Geometry check sheet. Reference: the model listing, model coordinates, mm. Face numbers are marked on the shaded views. A direction names the side the tool comes from. Round coordinates to 2 decimals unless told otherwise and drop trailing zeros. Write each loop counter-clockwise with the first axis right and the second up, starting at its lowest first coordinate (ties: lowest second). Pieces come first, ordered by that corner, then holes. Notation, with made-up numbers: (35.25, 54.25) - (83.25, 54.25) arc R10 cw to (83.25, 59.25) - close; hole circle Ø8 at (42, 16). An arc over 180 degrees is marked (long way). Return JSON: item names as keys, results as strings.
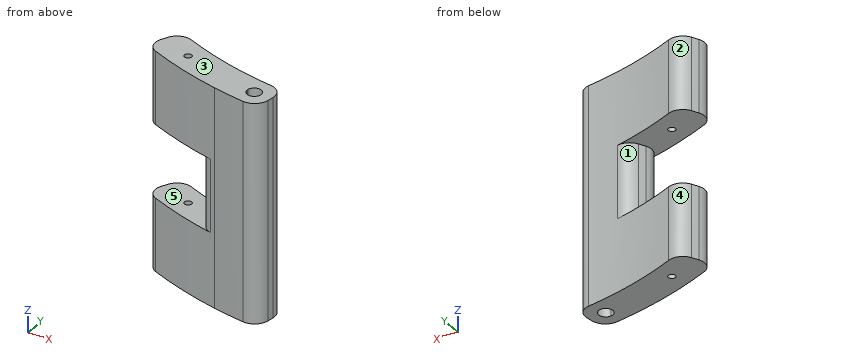
```python
from build123d import *

# Parameters (mm, degrees)
BOSS_EXTRUDE1_DEPTH     = 30
SKETCH2_W               = 10
SKETCH2_H               = 10
CUT_EXTRUDE2_DEPTH      = 37.330733855
SKETCH3_R               = 0.5
CUT_EXTRUDE3_DEPTH      = 30
FILLET1_R               = 2
SKETCH4_W               = 30
SKETCH4_H               = 5
BOSS_EXTRUDE2_DEPTH     = 10
FILLET2_R               = 2
FILLET3_R               = 2
CUT_EXTRUDE4_DEPTH      = 80.110177146
SKETCH6_W               = 10
SKETCH6_H               = 6
SKETCH8_W               = 10
SKETCH8_H               = 2.121165988
CUT_EXTRUDE5_DEPTH      = 80.110177146
FILLET4_R               = 8
CUT_EXTRUDE6_DEPTH      = 80.110177146
CUT_EXTRUDE6_DEPTH_BACK = 50
SCALE1_SCALE            = 1.9329
SCALE2_SCALE            = 1.5
CUT_EXTRUDE7_DEPTH      = 134.461525953
CUT_EXTRUDE7_DEPTH_BACK = 134.461525953
SKETCH10_R              = 280.344567012
SKETCH10_R_2            = 173.961
FILLET5_R               = 6


with BuildPart() as part:
    # Sketch1 → Boss-Extrude1 (new body)
    with BuildSketch(Plane.XY):
        with BuildLine():
            Line((-24.447759697, -49.267707941), (-26.670283306, -53.746590482))
            ThreePointArc((-26.670283306, -53.746590482), (-17.396934794, -57.422527459), (-7.642718065, -59.511249866))
            Line((-7.642718065, -59.511249866), (-7.005824893, -54.551979044))
            ThreePointArc((-7.005824893, -54.551979044), (-15.947190228, -52.637316837), (-24.447759697, -49.267707941))
        make_face()
    extrude(amount=BOSS_EXTRUDE1_DEPTH)

    # Sketch2 → Cut-Extrude2 (cut, through all)
    with BuildSketch(Plane(origin=(-26.670283306, -53.746590482, 0), x_dir=(0, 0, -1), z_dir=(0.4445047217595844, 0.8957765080272169, 0))):
        with Locations((-15, -5)):
            Rectangle(SKETCH2_W, SKETCH2_H)
    extrude(amount=CUT_EXTRUDE2_DEPTH, mode=Mode.SUBTRACT)

    # Sketch3 → Cut-Extrude3 (cut)
    with BuildSketch(Plane.XY.offset(30)):
        with Locations((-20.983324138, -53.534569281)):
            Circle(SKETCH3_R)
    extrude(amount=-CUT_EXTRUDE3_DEPTH, mode=Mode.SUBTRACT)

    # Fillet1
    fillet1_edges = [part.edges().sort_by_distance(p)[0] for p in [
        (-26.670283306, -53.746590482, 5),
        (-24.447759697, -49.267707941, 5),
        (-15.082503417, -52.891569183, 15),
        (-17.339488899, -57.439900111, 15),
        (-26.670283306, -53.746590482, 25),
        (-24.447759697, -49.267707941, 25),
    ]]
    fillet(fillet1_edges, radius=FILLET1_R)

    # Sketch4 → Boss-Extrude2 (add)
    with BuildSketch(Plane(origin=(-7.515339431, -58.519395701, 0), x_dir=(0, 0, -1), z_dir=(-0.12737863441697944, -0.9918541644284535, 0))):
        with Locations((-15, -2.5)):
            Rectangle(SKETCH4_W, SKETCH4_H)
    extrude(amount=BOSS_EXTRUDE2_DEPTH)

    # Fillet2
    fillet2_edges = [part.edges().sort_by_distance(p)[0] for p in [
        (-12.575405439, -58.667360415, 15),
    ]]
    fillet(fillet2_edges, radius=FILLET2_R)

    # Fillet3
    fillet3_edges = [part.edges().sort_by_distance(p)[0] for p in [
        (-7.005824893, -54.551979044, 15),
    ]]
    fillet(fillet3_edges, radius=FILLET3_R)

    # Sketch5 → Cut-Extrude4 (cut, through all)
    with BuildSketch(Plane.XY.offset(30)):
        with BuildLine():
            ThreePointArc((-10.9503146, -65.639855348), (-11.509930999, -66.072093113), (-11.077693234, -66.631709513))
            Line((-11.077693234, -66.631709513), (-10.9503146, -65.639855348))
        make_face()
        with BuildLine():
            Line((-10.9503146, -65.639855348), (-11.077693234, -66.631709513))
            ThreePointArc((-11.077693234, -66.631709513), (-10.683734829, -66.51117866), (-10.514003917, -66.135782431))
            ThreePointArc((-10.514003917, -66.135782431), (-10.638607687, -65.805513342), (-10.9503146, -65.639855348))
        make_face()
    extrude(amount=-CUT_EXTRUDE4_DEPTH, mode=Mode.SUBTRACT)

    # Cut-Sweep1: sweep along a path in Sketch7
    with BuildLine(Plane.XY) as cut_sweep1_path:
        Line((-8.024853968, -62.486812359), (-12.806249613, -60.46486559))
    # Sketch6 → Cut-Sweep1 (sweep, cut)
    with BuildSketch(Plane(origin=(0, 0, 0), x_dir=(0, 0, -1), z_dir=(0.9918541644284535, -0.1273786344169795, 0))):
        with Locations((-15, -66)):
            Rectangle(SKETCH6_W, SKETCH6_H)
    sweep(path=cut_sweep1_path.line, mode=Mode.SUBTRACT)

    # Sketch8 → Cut-Extrude5 (cut, through all)
    with BuildSketch(Plane(origin=(0, 0, 0), x_dir=(0, 0, -1), z_dir=(0.9918541644284535, -0.1273786344169795, 0))):
        with Locations((-15, -67.939417006)):
            Rectangle(SKETCH8_W, SKETCH8_H)
    extrude(amount=-CUT_EXTRUDE5_DEPTH, mode=Mode.SUBTRACT)

    # Fillet4
    fillet4_edges = [part.edges().sort_by_distance(p)[0] for p in [
        (-12.806249613, -60.46486559, 15),
    ]]
    fillet(fillet4_edges, radius=FILLET4_R)

    # Sketch9 → Cut-Extrude6 (cut, two sides: drawn at the far end of the back side and taken through both)
    with BuildSketch(Plane(origin=(0, 0, 0), x_dir=(-1, 0, 0), z_dir=(0, 0, -1)).offset(-CUT_EXTRUDE6_DEPTH_BACK)):
        with BuildLine():
            ThreePointArc((10.780840063, -56.480292913), (8.989884423, -56.068817625), (9.924359498, -57.651091416))
            Line((9.924359498, -57.651091416), (9.796980863, -56.659237252))
            ThreePointArc((9.796980863, -56.659237252), (10.28929948, -56.571903947), (10.780840063, -56.480292913))
        make_face()
        with BuildLine():
            Line((9.796980863, -56.659237252), (9.924359498, -57.651091416))
            ThreePointArc((9.924359498, -57.651091416), (10.547773323, -57.319775428), (10.796980863, -56.659237252))
            ThreePointArc((10.796980863, -56.659237252), (10.792937489, -56.569401844), (10.780840063, -56.480292913))
            ThreePointArc((10.780840063, -56.480292913), (10.28929948, -56.571903947), (9.796980863, -56.659237252))
        make_face()
    extrude(amount=CUT_EXTRUDE6_DEPTH + CUT_EXTRUDE6_DEPTH_BACK, mode=Mode.SUBTRACT)


with BuildPart() as part_1:
    # Scale1: scaled about (-14.187636467, -57.651950404, 15)
    add(part.part.scale(SCALE1_SCALE).moved(Location((13.23564606, 53.783504532, -13.9935))))


with BuildPart() as part_2:
    # Scale2: scaled about (-14.187636468, -57.651950404, 15)
    add(part_1.part.scale(SCALE2_SCALE).moved(Location((7.093818234, 28.825975202, -7.5))))

    # Sketch10 → Cut-Extrude7 (cut, two sides: drawn at the far end of the back side and taken through both)
    with BuildSketch(Plane.XY.offset(58.49025).offset(-CUT_EXTRUDE7_DEPTH_BACK)):
        with Locations((26.947287324, 109.501231999)):
            Circle(SKETCH10_R)
        with Locations((26.947287324, 109.501231999)):
            Circle(SKETCH10_R_2, mode=Mode.SUBTRACT)
    extrude(amount=CUT_EXTRUDE7_DEPTH + CUT_EXTRUDE7_DEPTH_BACK, mode=Mode.SUBTRACT)

    # Fillet5
    fillet5_edges = [part_2.edges().sort_by_distance(p)[0] for p in [
        (4.788372702, -63.042710299, 15),
    ]]
    fillet(fillet5_edges, radius=FILLET5_R)


solid = part_2.part
```
(1) Release check for a two-part mould opening along Z. For the marked faces 3, 4 and 5 record: pulls with the +Z half, pulls with the -Z half, needs draft (parallel to the pull), parting line crosses it, or undercut.
Response values:
{"face 3": "pulls with the +Z half", "face 4": "needs draft", "face 5": "undercut"}
(2) Section check C-C, the plane y = -55.75. Enter the section's corners in (x, z).
Response values:
{"outline": "(-27.41, -28.49) - (-4.19, -28.49) - (-4.19, 58.49) - (-27.41, 58.49) - (-27.41, 29.5) - (-20.29, 29.5) - (-20.29, 0.5) - (-27.41, 0.5) - close; (1.27, -28.49) - (5.72, -28.49) - (5.72, 58.49) - (1.27, 58.49) - close"}
(3) Material ranges on line 1 along Z through (x, y) = (-31, -39.75); line 2 along Y through (x, z) = (-14.5, 19); line 3 along X through (y, z) = (-57, 9.5) (3 decimals), recorded low to high. Write a range as [from, to].
Response values:
{"line 1": "z = [-28.49, 0.5], [29.5, 58.49]", "line 2": "y = [-59.45, -44.94]", "line 3": "x = [-19.516, -3.315], [0.4, 5.564]"}
(4) Section check A-A, the plane z = -19. Enter the section's corners in (x, y), plus the area to 3 significant figures.
Response values:
{"outline": "(-47.76, -41.05) arc R5.8 ccw to (-44.96, -48.9) arc R173.96 ccw to (-1.36, -62.14) arc R6 ccw to (5.57, -56.99) - (5.91, -54.31) arc R5.8 ccw to (1.1, -47.85) arc R159.46 cw to (-38.88, -35.74) arc R5.8 ccw to (-46.47, -38.45) - close; hole circle Ø2.9 at (-33.89, -45.71); hole circle Ø5.8 at (-1.46, -54.77)", "area": "742 mm^2"}
(5) Section check D-D, the plane z = 17.5. Enter the section's corners in (x, y), plus the area to 3 significant figures.
Response values:
{"outline": "(-20.21, -50.76) arc R5.8 ccw to (-16.47, -58.96) arc R173.96 ccw to (-1.36, -62.14) arc R6 ccw to (5.57, -56.99) - (5.91, -54.31) arc R5.8 ccw to (1.1, -47.85) arc R159.46 cw to (-12.27, -45.06) arc R5.8 ccw to (-18.89, -48.11) - close; hole circle Ø5.8 at (-1.46, -54.77)", "area": "325 mm^2"}
(6) Section check B-B, the plane x = -29. Enter the section's corners in (y, z), plus the area to 3 significant figures.
Response values:
{"outline": "(-55.22, -28.49) - (-39.83, -28.49) - (-39.83, 0.5) - (-55.22, 0.5) - close; (-55.22, 29.5) - (-39.83, 29.5) - (-39.83, 58.49) - (-55.22, 58.49) - close", "area": "892 mm^2"}
(7) Access from +Z, -Z, +X, -X, +Y, -Y to the whole of each face (thin tool, end or side, straight path). Record for the marked faces 1 and 2.
Response values:
{"face 1": "+Y", "face 2": "+Z, -Z, +Y"}
(8) Gauge pin test, flat ends, axial feed: pin 1 (3 mm diameter, centred on y = -48, z = -5, fed in from +X); pin 2 (8 mm diameter, centred on x = -37.5, z = 49.5, fed in from -Y); pin 3 (1 mm diameter, centred on x = -27, y = -38, fed in from -Z); pin 4 (6 mm diameter, centred on x = -6, z = -17, fed in from -Y). Record the tip position at first contact, or that the pin passes through.
Response values:
{"pin 1": "stops at x = 4.28", "pin 2": "stops at y = -53.62", "pin 3": "passes through", "pin 4": "stops at y = -61.86"}
